Design review of the part built by this model. Coordinates are the model's own, in mm. Round coordinates to 2 decimals unless told otherwise and drop trailing zeros. Write each loop counter-clockwise with the first axis right and the second up, starting at its lowest first coordinate (ties: lowest second). Pieces come first, ordered by that corner, then holes.
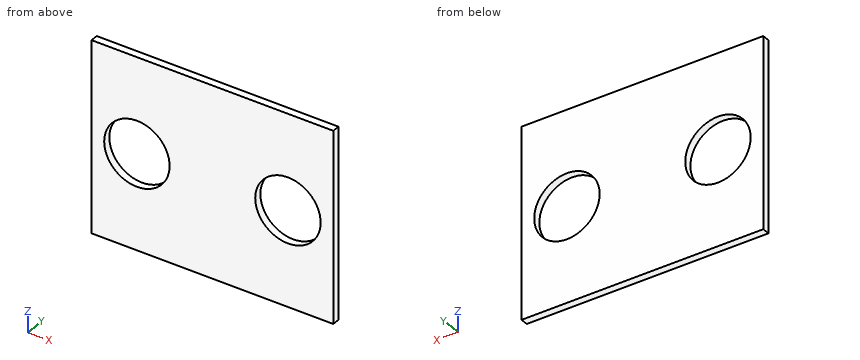
from build123d import *

# Parameters (mm, degrees)
F0_W     = 48
F0_H     = 38
F1_DEPTH = 1.5
F3_D     = 13
F3_DEPTH = 10


with BuildPart() as f1:
    # F0 (on Front) → F1 (new body)
    with BuildSketch(Plane.XZ):
        with Locations((24, 19)):
            Rectangle(F0_W, F0_H)
    extrude(amount=F1_DEPTH)

    # F3
    with Locations(Plane.XZ.offset(1.5)):
        with Locations((9, 19), (39, 19)):
            Hole(F3_D / 2, depth=F3_DEPTH)


solid = f1.part
1) Add section A-A on x = 41.5. State the section outline as (y, z) points.
2) For P1, Ø15, axis at x = 39, z = 19, coming from the -Y side, flat-tipped, find the tip position at first contact; note if it passes through.
3) Add section D-D on z = 15. State the section outline as (x, y) points.
4) For line 1 along Z through (x, y) = (39, -0.5); line 2 along X through (y, z) = (-0.7, 25); line 3 along X through (y, z) = (-1.2, 18.5), list the stretches that pass through material, from the lowest coordinate up.
5) Add section B-B on z = 19. State the section outline as (x, y) points.
6) Add section C-C on y = -0.6. State the section outline as (x, z) points.
Computed:
1. outline: (-1.5, 0) - (0, 0) - (0, 13) - (-1.5, 13) - close; (-1.5, 25) - (0, 25) - (0, 38) - (-1.5, 38) - close
2. P1: stops at y = -1.5
3. outline: (0, -1.5) - (3.88, -1.5) - (3.88, 0) - (0, 0) - close; (14.12, -1.5) - (33.88, -1.5) - (33.88, 0) - (14.12, 0) - close; (44.12, -1.5) - (48, -1.5) - (48, 0) - (44.12, 0) - close
4. line 1: z = 0 to 12.5, 25.5 to 38
4. line 2: x = 0 to 6.5, 11.5 to 36.5, 41.5 to 48
4. line 3: x = 0 to 2.52, 15.48 to 32.52, 45.48 to 48
5. outline: (0, -1.5) - (2.5, -1.5) - (2.5, 0) - (0, 0) - close; (15.5, -1.5) - (32.5, -1.5) - (32.5, 0) - (15.5, 0) - close; (45.5, -1.5) - (48, -1.5) - (48, 0) - (45.5, 0) - close
6. outline: (0, 0) - (48, 0) - (48, 38) - (0, 38) - close; hole circle Ø13 at (9, 19); hole circle Ø13 at (39, 19)
